Could you check a few things on this model? Use its own coordinates, in mm. Face numbers are marked on the shaded views. Give positions to 0.01 mm unless a question says otherwise; leave off trailing zeros. Order: outer loops, then holes, each group sorted by start corner. A loop starts at its lowest first (then second) coordinate and runs counter-clockwise, first axis right, second up. Notation, with made-up numbers: M -14,74.5 L -3,74.5 A13 cw -3,96.5 Z; hole C -21,-5.75 d4. An arc over 180 degrees is marked long. Use a Markdown table: item, result. Add a question column.
Item 1: I'm going to push a flat-ended pin straight in: pin 1 Ø2 at (y, z) = (7, -1.5) entering from -X. Where does the tip first touch, or does it pass through?
Item 2: Suppose I cut it at C-C on y = -10.5. Write out the boundary of the cut face in (x, z), plus the area to 3 significant figures.
Item 3: Suppose I cut it at B-B on z = -0.75. Write out the boundary of the cut face in (x, y), plus the area to 3 significant figures.
Item 4: If we mould it in two halves opening along Z, with no side actions, what happens to the marked faces 1 and 2? For each: released by +Z, released by -Z, zero draft, split by the parting line, or undercut.
Item 5: If I drill on L1, parallel to Y at x = -8.5, z = 1; L2, parallel to Y at x = -8.75, z = 2.5; L3, parallel to X at y = 21, z = -2, over which ranges is the centre line in solid material (lowest first)? Write a range as from..to.
Item 6: Suppose I cut it at A-A on x = 8.25. Write out the boundary of the cut face in (y, z).
from build123d import *

# Parameters (mm, degrees)
SKETCH1_W           = 19.999999878
SKETCH1_H           = 200.00000005
BOSS_EXTRUDE1_DEPTH = 3.499999985
CUT_EXTRUDE1_DEPTH  = 7.112


with BuildPart() as part:
    # Sketch1 → Boss-Extrude1 (new, symmetric)
    with BuildSketch(Plane.XY):
        Rectangle(SKETCH1_W, SKETCH1_H)
    extrude(amount=BOSS_EXTRUDE1_DEPTH, both=True)

    # Sketch2 → Cut-Extrude1 (cut)
    with BuildSketch(Plane.XY.offset(3.499999985)):
        with BuildLine():
            ThreePointArc((-9.999999939, 19.57321454), (-7.225569373, 23.658770866), (-6.249999946, 28.500000023))
            ThreePointArc((-6.249999946, 28.500000023), (-7.225569373, 33.34122918), (-9.999999939, 37.426785506))
            Line((-9.999999939, 37.426785506), (-9.999999939, 19.57321454))
        make_face()
        with BuildLine():
            ThreePointArc((-9.999999939, 37.426785506), (-31.24999973, 28.500000023), (-9.999999939, 19.57321454))
            Line((-9.999999939, 19.57321454), (-9.999999939, 37.426785506))
        make_face()
        with BuildLine():
            ThreePointArc((9.999999939, 37.426785506), (7.225569373, 33.34122918), (6.249999946, 28.500000023))
            ThreePointArc((6.249999946, 28.500000023), (7.225569373, 23.658770866), (9.999999939, 19.57321454))
            Line((9.999999939, 19.57321454), (9.999999939, 37.426785506))
        make_face()
        with BuildLine():
            Line((9.999999939, 37.426785506), (9.999999939, 19.57321454))
            ThreePointArc((9.999999939, 19.57321454), (23.591228995, 16.975569558), (31.24999973, 28.500000023))
            ThreePointArc((31.24999973, 28.500000023), (23.591228995, 40.024430488), (9.999999939, 37.426785506))
        make_face()
        with BuildLine():
            Line((6.249999946, 28.500000023), (6.249999946, -28.500000023))
            ThreePointArc((6.249999946, -28.500000023), (7.225569373, -23.658770866), (9.999999939, -19.57321454))
            Line((9.999999939, -19.57321454), (9.999999939, 19.57321454))
            ThreePointArc((9.999999939, 19.57321454), (7.225569373, 23.658770866), (6.249999946, 28.500000023))
        make_face()
        with BuildLine():
            ThreePointArc((-9.999999939, -19.57321454), (-7.225569373, -23.658770866), (-6.249999946, -28.500000023))
            Line((-6.249999946, -28.500000023), (-6.249999946, 28.500000023))
            ThreePointArc((-6.249999946, 28.500000023), (-7.225569373, 23.658770866), (-9.999999939, 19.57321454))
            Line((-9.999999939, 19.57321454), (-9.999999939, -19.57321454))
        make_face()
        with BuildLine():
            ThreePointArc((-9.999999939, -37.426785506), (-7.225569373, -33.34122918), (-6.249999946, -28.500000023))
            ThreePointArc((-6.249999946, -28.500000023), (-7.225569373, -23.658770866), (-9.999999939, -19.57321454))
            Line((-9.999999939, -19.57321454), (-9.999999939, -37.426785506))
        make_face()
        with BuildLine():
            Line((-9.999999939, -37.426785506), (-9.999999939, -19.57321454))
            ThreePointArc((-9.999999939, -19.57321454), (-31.24999973, -28.500000023), (-9.999999939, -37.426785506))
        make_face()
        with BuildLine():
            ThreePointArc((9.999999939, -19.57321454), (7.225569373, -23.658770866), (6.249999946, -28.500000023))
            ThreePointArc((6.249999946, -28.500000023), (7.225569373, -33.34122918), (9.999999939, -37.426785506))
            Line((9.999999939, -37.426785506), (9.999999939, -19.57321454))
        make_face()
        with BuildLine():
            ThreePointArc((31.24999973, -28.500000023), (23.591228995, -16.975569558), (9.999999939, -19.57321454))
            Line((9.999999939, -19.57321454), (9.999999939, -37.426785506))
            ThreePointArc((9.999999939, -37.426785506), (23.591228995, -40.024430488), (31.24999973, -28.500000023))
        make_face()
    extrude(amount=-CUT_EXTRUDE1_DEPTH, mode=Mode.SUBTRACT)


solid = part.part
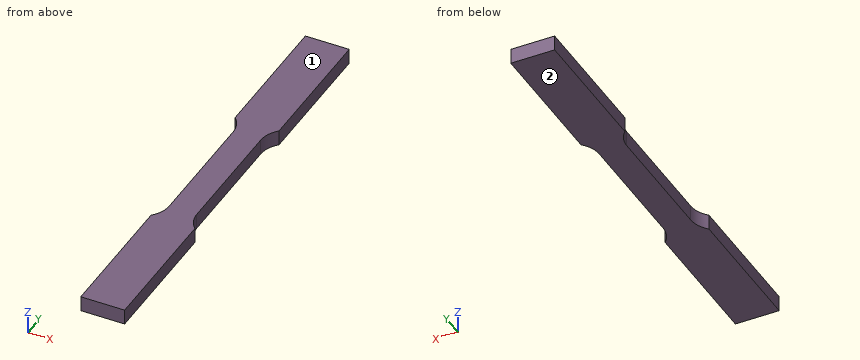
Findings below:
| question | item | result |
|---|---|---|
| 1 | pin 1 | stops at x = -6.25 |
| 2 | outline | M -6.25,-3.5 L 6.25,-3.5 L 6.25,3.5 L -6.25,3.5 Z |
| 2 | area | 87.5 mm^2 |
| 3 | outline | M -10,-100 L 10,-100 L 10,-37.43 A12.5 cw 6.25,-28.5 L 6.25,28.5 A12.5 cw 10,37.43 L 10,100 L -10,100 L -10,37.43 A12.5 cw -6.25,28.5 L -6.25,-28.5 A12.5 cw -10,-37.43 Z |
| 3 | area | 3,480 mm^2 |
| 4 | face 1 | released by +Z |
| 4 | face 2 | released by -Z |
| 5 | L1 | y = -100..-35.65, 35.65..100 |
| 5 | L2 | y = -100..-36, 36..100 |
| 5 | L3 | x = -6.25..6.25 |
| 6 | outline | M -100,-3.5 L -35.28,-3.5 L -35.28,3.5 L -100,3.5 Z; M 35.28,-3.5 L 100,-3.5 L 100,3.5 L 35.28,3.5 Z |
